Part model, mm, in its own coordinate system. Face numbers are marked on the shaded views. A direction names the side the tool comes from. Round coordinates to 2 decimals unless told otherwise and drop trailing zeros. Order: outer loops, then holes, each group sorted by start corner. A loop starts at its lowest first (then second) coordinate and runs counter-clockwise, first axis right, second up. Notation, with made-up numbers: (31, 73) -> (48, 73) arc R23 ccw to (48, 92) -> close; hole circle Ø2 at (79, 56). An arc over 180 degrees is marked (long way). Use CSV: the item, a comma, the result in double quotes.
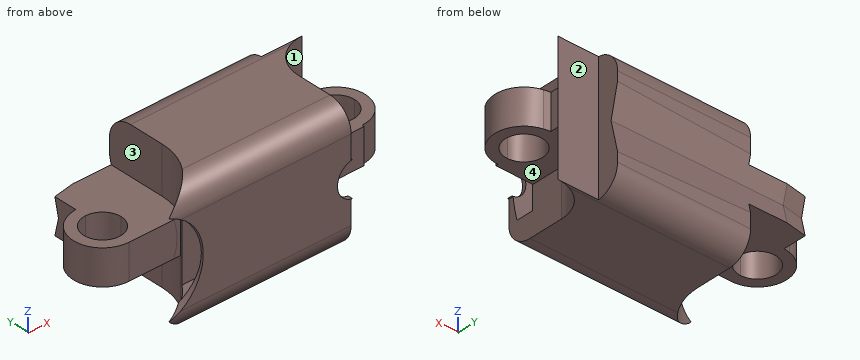
```python
from build123d import *
from build123d.topology import SkipClean

# Parameters (mm, degrees)
SKETCH1_R               = 1.6
BOSS_EXTRUDE1_DEPTH     = 1.5
SKETCH2_W               = 18
SKETCH2_H               = 5
BOSS_EXTRUDE3_DEPTH     = 20
CUT_EXTRUDE3_DEPTH      = 4
CUT_EXTRUDE1_DEPTH      = 4
CUT_EXTRUDE4_DEPTH      = 6
CUT_EXTRUDE5_DEPTH      = 25.088378991
CUT_EXTRUDE5_DEPTH_BACK = 25.088378991
SKETCH11_R              = 1.6
CUT_EXTRUDE6_DEPTH      = 10
SKETCH13_R              = 4.127392351
CUT_EXTRUDE7_DEPTH      = 2.5
CUT_EXTRUDE8_START      = -3.5
CUT_EXTRUDE8_DEPTH      = 3.5


with BuildPart() as part:
    # Sketch1 → Boss-Extrude1 (new, symmetric)
    with BuildSketch(Plane.XY):
        with BuildLine():
            Line((0, -2.5), (20, -2.5))
            ThreePointArc((20, -2.5), (22.485953156, -0.264644865), (20.526315789, 2.443970476))
            ThreePointArc((20.526315789, 2.443970476), (10, 3.564560947), (-0.526315789, 2.443970476))
            ThreePointArc((-0.526315789, 2.443970476), (-2.485953156, -0.264644865), (0, -2.5))
        make_face()
        Circle(SKETCH1_R, mode=Mode.SUBTRACT)
        with Locations((20, 0)):
            Circle(SKETCH1_R, mode=Mode.SUBTRACT)
    extrude(amount=BOSS_EXTRUDE1_DEPTH, both=True)

    # Sketch2 → Revolve1 (revolve)
    with BuildSketch(Plane(origin=(0, 0, 0), x_dir=(1, 0, 0), z_dir=(0, 1, 0))):
        with Locations((11, -2.5)):
            Rectangle(SKETCH2_W, SKETCH2_H)
    revolve(axis=Axis((2, 0, 0), (1, 0, 0)))

    # Sketch9 → Boss-Extrude3 (add)
    with BuildSketch(Plane(origin=(0, 0, 0), x_dir=(0, 0, -1), z_dir=(1, 0, 0))):
        with BuildLine():
            Line((-3.5, -5), (3.5, -5))
            ThreePointArc((3.5, -5), (4.914213562, -4.414213562), (5.5, -3))
            Line((5.5, -3), (5.5, 3))
            ThreePointArc((5.5, 3), (4.914213562, 4.414213562), (3.5, 5))
            Line((3.5, 5), (-3.5, 5))
            ThreePointArc((-3.5, 5), (-4.914213562, 4.414213562), (-5.5, 3))
            Line((-5.5, 3), (-5.5, -3))
            ThreePointArc((-5.5, -3), (-4.914213562, -4.414213562), (-3.5, -5))
        make_face()
    extrude(amount=BOSS_EXTRUDE3_DEPTH)

    # Cut-Sweep1: sweep along a path in Sketch4
    with BuildLine(Plane.XY) as cut_sweep1_path:
        Line((24.863277649, 2.710997103), (2, 2.920411664))
        ThreePointArc((2, 2.920411664), (0.733779453, 2.698430699), (-0.526315789, 2.443970476))
        Line((-0.526315789, 2.443970476), (-4.067756882, 1.923712717))
    # Sketch3 → Cut-Sweep1 (sweep, cut)
    with BuildSketch(Plane(origin=(0, 0, 0), x_dir=(0, 0, -1), z_dir=(1, 0, 0))):
        Polygon((3.5, 5), (0, 4.182726474), (-3.5, 5), (-3.5, 6.035180102), (3.681581058, 6.035180102), align=None)
    sweep(path=cut_sweep1_path.line, transition=Transition.RIGHT, mode=Mode.SUBTRACT)

    # Cut-Sweep3: sweep along a path in Sketch7
    with BuildLine(Plane.XY) as cut_sweep3_path:
        Line((0, -2.91172129), (20, -2.693253741))
    # Sketch6 → Cut-Sweep3 (sweep, cut)
    with BuildSketch(Plane(origin=(20, 0, 0), x_dir=(0, 0, -1), z_dir=(1, 0, 0))):
        with BuildLine():
            Line((3.5, -2.693253741), (3.5, -4.193253741))
            ThreePointArc((3.5, -4.193253741), (0, -4.643536391), (-3.5, -4.193253741))
            Line((-3.5, -4.193253741), (-3.5, -2.693253741))
            Line((-3.5, -2.693253741), (3.5, -2.693253741))
        make_face()
    sweep(path=cut_sweep3_path.line, mode=Mode.SUBTRACT)

    # Sketch8 → Cut-Extrude3 (cut)
    with BuildSketch(Plane.XY.offset(1.5)):
        with BuildLine():
            Line((16.8, 0), (16.8, -2))
            Line((16.8, -2), (16.8, -5))
            Line((16.8, -5), (20, -5))
            Line((20, -5), (20, -3.2))
            ThreePointArc((20, -3.2), (22.2627417, 2.2627417), (16.8, 0))
        make_face()
    cut_extrude3 = extrude(amount=CUT_EXTRUDE3_DEPTH, mode=Mode.SUBTRACT)

    # Sketch5 → Cut-Extrude1 (cut)
    with BuildSketch(Plane.XY.offset(1.5)):
        with BuildLine():
            Line((5.1, 0), (5.1, 5.1))
            Line((5.1, 5.1), (0, 5.1))
            ThreePointArc((0, 5.1), (-3.606244584, -3.606244584), (5.1, 0))
        make_face()
    cut_extrude1 = extrude(amount=CUT_EXTRUDE1_DEPTH, mode=Mode.SUBTRACT)

    # Mirror1: Cut-Extrude3, Cut-Extrude1 across plane
    add(cut_extrude3.mirror(Plane.XY), mode=Mode.SUBTRACT)
    add(cut_extrude1.mirror(Plane.XY), mode=Mode.SUBTRACT)

    # Sketch10 → Cut-Extrude4 (cut)
    with BuildSketch(Plane(origin=(0.031802036, -2.911373904, 0), x_dir=(0.9999403452508379, 0.01092272583357663, 0), z_dir=(0.01092272583357663, -0.9999403452508379, 0))):
        with BuildLine():
            Line((17.174273437, 1.517261574), (23.592478812, 1.517261574))
            Line((23.592478812, 1.517261574), (23.592478812, -1.517261574))
            Line((23.592478812, -1.517261574), (17.174357812, -1.517261574))
            Line((17.174357812, -1.517261574), (17.08845436, -1.517261574))
            ThreePointArc((17.08845436, -1.517261574), (15.571192786, 0), (17.08845436, 1.517261574))
            Line((17.08845436, 1.517261574), (17.174273437, 1.517261574))
        make_face()
    extrude(amount=CUT_EXTRUDE4_DEPTH, mode=Mode.SUBTRACT)

    # Sketch11 → Cut-Extrude5 (cut, two sides: drawn at the far end of the back side and taken through both)
    with SkipClean():  # the faces are left unmerged after this step: merging them gives an invalid solid
        with BuildSketch(Plane.XY.offset(1.5).offset(-CUT_EXTRUDE5_DEPTH_BACK)):
            with Locations((20, 0)):
                Circle(SKETCH11_R)
            Circle(SKETCH11_R)
        extrude(amount=CUT_EXTRUDE5_DEPTH + CUT_EXTRUDE5_DEPTH_BACK, mode=Mode.SUBTRACT)

    # Sketch12 → Cut-Extrude6 (cut)
    with SkipClean():  # the faces are left unmerged after this step: merging them gives an invalid solid
        with BuildSketch(Plane.XY.offset(1.5)):
            with BuildLine():
                Line((2, -2.5), (4.445222154, -2.5))
                ThreePointArc((4.445222154, -2.5), (2.659498662, -4.35167403), (0.197141337, -5.09618831))
                Line((0.197141337, -5.09618831), (-0.979949821, -5.09618831))
                Line((-0.979949821, -5.09618831), (-0.979949821, -2.5))
                Line((-0.979949821, -2.5), (2, -2.5))
            make_face()
        extrude(amount=-CUT_EXTRUDE6_DEPTH, mode=Mode.SUBTRACT)

    # Sketch13 → Cut-Extrude7 (cut)
    with BuildSketch(Plane.XZ.offset(5)):
        Circle(SKETCH13_R)
    extrude(amount=-CUT_EXTRUDE7_DEPTH, mode=Mode.SUBTRACT)

    # Sketch15 → Cut-Extrude8 (cut)
    with BuildSketch(Plane(origin=(20, 0, 0), x_dir=(0, 0, -1), z_dir=(1, 0, 0)).offset(CUT_EXTRUDE8_START)):
        with BuildLine():
            Line((-2.836208081, 5), (2.836208081, 5))
            Line((2.836208081, 5), (3.5, 5))
            ThreePointArc((3.5, 5), (4.841640786, 4.483239697), (5.489974874, 3.2))
            Line((5.489974874, 3.2), (1.5, 3.2))
            Line((1.5, 3.2), (-1.5, 3.2))
            Line((-1.5, 3.2), (-5.489974874, 3.2))
            ThreePointArc((-5.489974874, 3.2), (-4.841640786, 4.483239697), (-3.5, 5))
            Line((-3.5, 5), (-2.836208081, 5))
        make_face()
    extrude(amount=CUT_EXTRUDE8_DEPTH, mode=Mode.SUBTRACT)


solid = part.part
```
(1) Cut at A-A, the plane x = 19.25. Give the cut face in (y, z), then the cut area to 3 significant figures.
Reply:
outline,"(-2.7, -1.5) -> (-1.41, -1.5) -> (-1.41, 1.5) -> (-2.7, 1.5) -> close; (1.41, -1.5) -> (3.11, -1.5) -> (3.11, -5.5) arc R2 ccw to (3.2, -5.49) -> (3.2, 5.49) arc R2 ccw to (3.11, 5.5) -> (3.11, 1.5) -> (1.41, 1.5) -> close"
area,"9.94 mm2"
(2) Probe probe 1 along Z at (x, y) = (8, -3.25); probe 2 along X at (y, z) = (0.75, -1.25); probe 3 along X at (y, z) = (-2.5, -2.5). List the from-to ranges inside material, lowest first. Write a range as [from, to].
Reply:
probe 1,"[-5.48, -3.5], [3.5, 5.48]"
probe 2,"[-2.38, -1.41], [1.41, 18.59], [21.41, 22.38]"
probe 3,"[4.45, 16.8]"
(3) Cut at B-B, the plane z = 5.25. Give the cut face in (x, y), then the cut area to 3 significant figures.
Reply:
outline,"(3.2, -3.97) -> (16.8, -3.97) -> (16.8, 0) arc R3.2 cw to (20, 3.2) -> (16.5, 3.2) -> (16.5, 3.97) -> (5.1, 3.97) -> (5.1, 0) arc R5.1 cw to start"
area,"97.1 mm2"
(4) Drop flat-ended pins along their axis: P1, Ø3.5, axis at x = 0, y = 0, coming from the +Z side; P2, Ø0.6, axis at y = 3.5, z = 0, coming from the -X side; P3, Ø3, axis at y = -1.5, z = 2.5, coming from the +X side. Give the stop position or say it passes through.
Reply:
P1,"z = 1.5"
P2,"x = 0"
P3,"x = 22.47"
(5) Which spindle directions (+Z, -Z, +X, -X, +Y, -Y) get a long thin tool onto all of the face, cutting with end or side? Do the marked faces 1, 2, 3 and 4. Say none if no direction does.
Reply:
face 1,"+Z, +X, -Y"
face 2,"+Z, -Z, +X, +Y"
face 3,"+Z, -X, +Y"
face 4,"-Z, +X, -Y"
